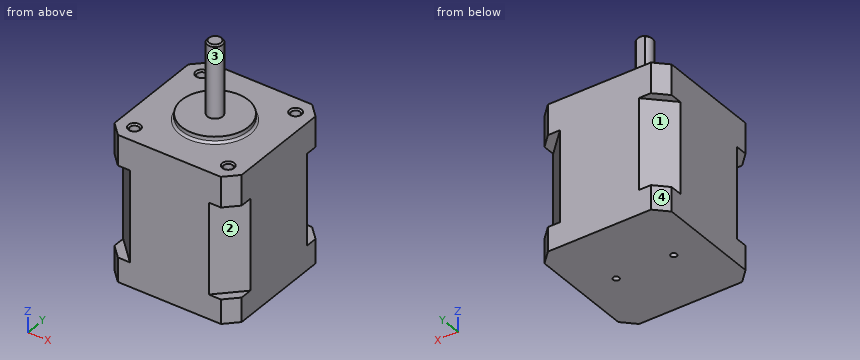
Autodesk Inventor part; units mm, degrees
ref_plane "YZ Plane" through (0, 0, 0) normal (1, 0, 0) x (0, 1, 0)
ref_plane "XZ Plane" through (0, 0, 0) normal (0, 1, 0) x (-1, 0, 0)
ref_plane "XY Plane" through (0, 0, 0) normal (0, 0, 1) x (1, 0, 0)
sketch "Sketch1" plane through (0, 0, 0) normal (0, 0, 1) x (1, 0, 0)
  line L0 (21, 42) -> (-21, 42)
  line L1 (-21, 42) -> (-21, 0)
  line L2 (-21, 0) -> (21, 0)
  line L3 (21, 0) -> (21, 42)
  point P0 (0, 0)
  point P1 (0, 0)
  dimension "d0" = 42
  dimension "d1" = 42
extrude "Extrusion1" add sketch "Sketch1" along normal blind 48
ref_plane "Work Plane1" through (0, 0, 38) normal (0, 0, 1) x (1, 0, 0)
sketch "Sketch2" plane through (0, 0, 38) normal (0, 0, 1) x (1, 0, 0)
  line L0 (21, 42) -> (-21, 42)
  line L1 (-21, 42) -> (-21, 0)
  line L2 (-21, 0) -> (21, 0)
  line L3 (21, 0) -> (21, 42)
  line L4 (-21, 42) -> (-21, 0)
  line L5 (-21, 34) -> (-13, 42)
  line L6 (21, 42) -> (-21, 42)
  line L7 (0, 50.0167) -> (0, -8.0167)
  line L8 (-21, 21) -> (21, 21)
  line L9 (21, 34) -> (13, 42)
  line L10 (-21, 8) -> (-13, 0)
  line L11 (21, 8) -> (13, 0)
  line L12 (-21, 34) -> (-21, 42)
  line L13 (-13, 42) -> (-21, 42)
  line L14 (13, 42) -> (21, 42)
  line L15 (21, 42) -> (21, 34)
  line L16 (21, 8) -> (21, 0)
  line L17 (21, 0) -> (21, 42)
  line L18 (-21, 0) -> (21, 0)
  line L19 (21, 0) -> (13, 0)
  line L20 (-13, 0) -> (-21, 0)
  line L21 (-21, 0) -> (-21, 8)
  point P0 (0, 0)
  point P1 (0, 21)
  dimension "d5" = 8
  dimension "d6" = 8
  dimension "d7" = 42
extrude "Extrusion2" cut sketch "Sketch2" against normal blind 30 contours L3 L9 L0 | L5 L1 L0 | L3 L2 L11 | L2 L1 L10
chamfer "Chamfer1" distance 4 angle 45 8 edges at (-21, 42, 43) (21, 42, 43) (21, 0, 43) (-21, 0, 43) (-21, 42, 4) (21, 42, 4) (-21, 0, 4) (21, 0, 4)
sketch "Sketch3" plane through (0, 0, 48) normal (0, 0, 1) x (1, 0, 0)
  line L0 (21, 38) -> (21, 4)
  line L1 (-17, 42) -> (17, 42)
  line L2 (-21, 4) -> (-21, 38)
  line L3 (0, 42) -> (0, 0)
  line L4 (-21, 21) -> (21, 21)
  point P0 (-15.5, 5.5)
  point P1 (15.5, 5.5)
  point P2 (-15.5, 36.5)
  point P3 (15.5, 36.5)
  dimension "d13" = 31
  dimension "d14" = 31
hole "Hole1" at (-15.5, 5.5, 48) at (15.5, 5.5, 48) at (-15.5, 36.5, 48) at (15.5, 36.5, 48) direction (0, 0, -1) diameter 3 depth 4.5 tip angle 118 countersink diameter 4 countersink angle 90
sketch "Sketch5" plane through (0, 0, 0) normal (0, 0, -1) x (-1, 0, 0)
  line L0 (17, 0) -> (-17, 0)
  line L1 (17, 42) -> (-17, 42)
  line L2 (0, 42) -> (0, 0)
  point P0 (-9.5, 21)
  point P1 (9.5, 21)
  dimension "d28" = 19
hole "Hole2" at (9.5, 21, 0) at (-9.5, 21, 0) direction (0, 0, 1) diameter 2 depth 5.1 tip angle 118
sketch "Sketch6" plane through (0, 0, 48) normal (0, 0, 1) x (1, 0, 0)
  line L0 (-17, 42) -> (17, 42)
  line L1 (-21, 4) -> (-21, 38)
  line L2 (0, 42) -> (0, 0)
  circle A0 centre (0, 21) radius 11
  dimension "d36" = 22
extrude "Extrusion4" add sketch "Sketch6" along normal blind 2.03
fillet "Fillet1" radius 0.7 1 edges at (-11, 21, 48)
sketch "Sketch7" plane through (0, 21, 50.03) normal (0, 0, 1) x (1, 0, 0)
  circle A0 centre (0, 0) radius 11
  circle A1 centre (0, 0) radius 2.5
  point P0 (0, -21)
  dimension "d40" = 5
extrude "Extrusion5" add sketch "Sketch7" along normal blind 23.88 contours A1
sketch "Sketch8" plane through (0, 21, 73.91) normal (0, 0, 1) x (1, 0, 0)
  line L0 (-1.473, 2.02) -> (1.473, 2.02)
  circle A0 centre (0, 0) radius 2.5
  circle A1 centre (0, 0) radius 2.5
  circle A2 centre (0, 0) radius 2.5
  arc A3 (1.473, 2.02) -> (-1.473, 2.02) centre (0, 0) ccw
  point P0 (0, -21)
extrude "Extrusion6" cut sketch "Sketch8" against normal blind 14.86 contours A0 L0 picked at (0.3249, 2.2492)
chamfer "Chamfer2" distance 0.5 angle 45 2 edges at (-1.1331, 18.7715, 73.91) (2.2285, 22.1331, 73.91)
properties part number "nema 17 stepper motor (triple stack)"
Input: part model. Units: mm. Frame: model coordinates. Face numbers are marked on the shaded views. A direction names the side the tool comes from. Give positions to 0.01 mm unless a question says otherwise; leave off trailing zeros. Order: outer loops, then holes, each group sorted by start corner. A loop starts at its lowest first (then second) coordinate and runs counter-clockwise, first axis right, second up. Notation, with made-up numbers: (46, 29.25) - (77, 29.25) arc R18 ccw to (77, 46.25) - close; hole circle Ø6 at (16, 3). An arc over 180 degrees is marked (long way). Answer as a JSON object with one key per item and string values. Group by question number.
Q1. Line query: probe 1 along X at (y, z) = (21, 3.65); probe 2 along Y at (x, z) = (-15.5, 46.7); probe 3 along X at (y, z) = (5.5, 46.1). Output: solid intervals per line, ascending.
Q2. Cut plane A-A, the plane z = 19. Output: boundary loops of the cut face in (x, y).
Q3. First-contact query: pin 1 Ø9 at (x, y) = (-16.5, 4.5) entering from +Z; pin 2 Ø1.8 at (x, y) = (15.5, 36.5) entering from +Z; pin 3 Ø21 at (x, y) = (10.5, 28) entering from +Z. Flat tips, straight axial feed; report the tip coordinate or a pass-through.
Q4. Cut plane B-B, the plane z = 65. Output: boundary loops of the cut face in (x, y), then the cut area to 3 significant figures.
Q5. Cut plane C-C, the plane z = 54. Output: boundary loops of the cut face in (x, y), then the cut area to 3 significant figures.
Q6. Set-up query: the marked faces 1, 2, 3 and 4. Return all of +Z, -Z, +X, -X, +Y, -Y with unobstructed straight access to the full face (end or side cutting, diameter ignored); none if empty.
Results:
{
 "1": {"probe 1": "-21 to -10.5, -8.5 to 8.5, 10.5 to 21", "probe 2": "0 to 4, 7 to 35, 38 to 42", "probe 3": "-21 to -17, -14 to 14, 17 to 21"},
 "2": {"outline": "(-21, 8) - (-13, 0) - (13, 0) - (21, 8) - (21, 34) - (13, 42) - (-13, 42) - (-21, 34) - close"},
 "3": {"pin 1": "z = 48", "pin 2": "z = 43.14", "pin 3": "z = 73.79"},
 "4": {"outline": "(-1.47, 23.02) arc R2.5 ccw (long way) to (1.47, 23.02) - close", "area": "18.7 mm^2"},
 "5": {"outline": "circle Ø5 at (0, 21)", "area": "19.6 mm^2"},
 "6": {"face 1": "-X, +Y", "face 2": "+X, -Y", "face 3": "+Z", "face 4": "+Z, -Z, -X, +Y"}
}
